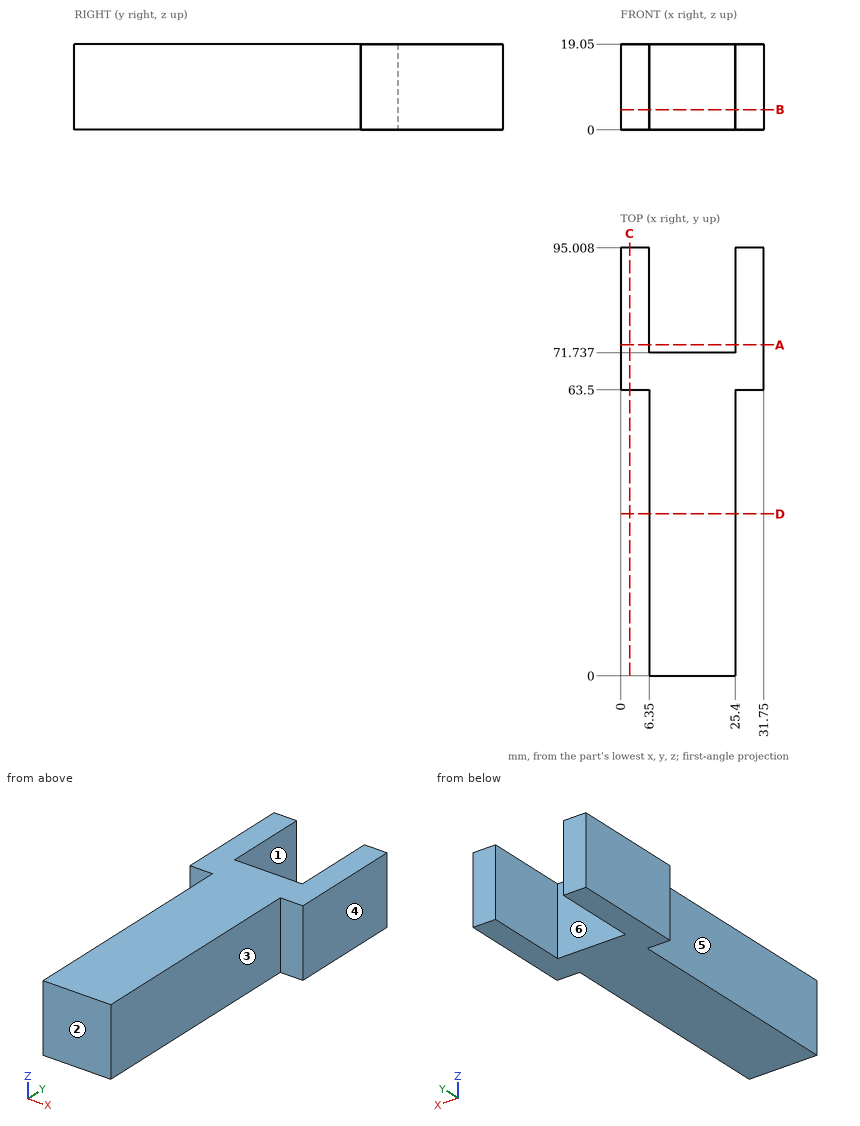
Could you check a few things on this drawing? It's one solid part, dimensions in mm from its lowest x, y, z. A direction names the side the tool comes from. Coordinates: 2 decimals unless noted, no trailing zeros. Order: outer loops, then holes, each group sorted by start corner. A loop starts at its lowest first (then second) coordinate and runs counter-clockwise, first axis right, second up. Notation, with made-up numbers: M 79,42.5 L 92,42.5 A30 ccw 92,65.5 Z; hole C 65,-7.5 d4. An arc over 180 degrees is marked long. Answer as a JSON object with one key per item and string values. Group by question number.
(1) Suppose I cut it at A-A, the plane y = 73.5. Please give me the cut outline in (x, z).
(2) I need wall thicknesses on probe 1 along X at (y, z) = (79, 13.25); probe 2 along Y at (x, z) = (21, 9.25); probe 3 along X at (y, z) = (7.5, 8). Which ranges of each line are inside material? Lowest first, please.
(3) Suppose I cut it at C-C, the plane x = 2. Please give me the cut outline in (y, z).
(4) Suppose I cut it at D-D, the plane y = 36. Please give me the cut outline in (x, z), then the cut area to 3 significant figures.
(5) If we mould it in two halves opening along X, with no side actions, what happens to the marked faces 4, 5 and 6? For each: released by +X, released by -X, zero draft, split by the parting line, or undercut.
(6) For pin 1 (1.5 mm diameter, centred on x = 20, z = 10, fed in from +Y); pin 2 (10 mm diameter, centred on y = 50.5, z = 8, fed in from -X); pin 3 (7 mm diameter, centred on x = 2, z = 6.5, fed in from -Y), each with a flat end and sliding along its axis, tell me the tip position at first contact or that it passes through.
(7) Which directions (+Z, -Z, +X, -X, +Y, -Y) give clear straight access to the entire face, cutting with the end or side of a thin tool? Please do the marked faces 1, 2 and 3.
(8) Suppose I cut it at B-B, the plane z = 4.5. Please give me the cut outline in (x, y).
Values found:
{
 "1": {"outline": "M 0,0 L 6.35,0 L 6.35,19.05 L 0,19.05 Z; M 25.4,0 L 31.75,0 L 31.75,19.05 L 25.4,19.05 Z"},
 "2": {"probe 1": "x = 0 to 6.35, 25.4 to 31.75", "probe 2": "y = 0 to 71.74", "probe 3": "x = 6.35 to 25.4"},
 "3": {"outline": "M 63.5,0 L 95.01,0 L 95.01,19.05 L 63.5,19.05 Z"},
 "4": {"outline": "M 6.35,0 L 25.4,0 L 25.4,19.05 L 6.35,19.05 Z", "area": "363 mm^2"},
 "5": {"face 4": "released by +X", "face 5": "released by -X", "face 6": "undercut"},
 "6": {"pin 1": "stops at y = 71.74", "pin 2": "stops at x = 6.35", "pin 3": "stops at y = 63.5"},
 "7": {"face 1": "+Z, -Z, +Y", "face 2": "+Z, -Z, +X, -X, -Y", "face 3": "+Z, -Z, +X, -Y"},
 "8": {"outline": "M 0,63.5 L 6.35,63.5 L 6.35,0 L 25.4,0 L 25.4,63.5 L 31.75,63.5 L 31.75,95.01 L 25.4,95.01 L 25.4,71.74 L 6.35,71.74 L 6.35,95.01 L 0,95.01 Z"}
}
